Could you check a few things on this model? Use its own coordinates, in mm. Give positions to 0.01 mm unless a question says otherwise; leave off trailing zeros. Loops run counter-clockwise (first coordinate to the right, second up) from the corner with the lowest first, then second, coordinate; pieces in that order, holes last. Notation, with made-up numbers: (-33.5, 18.5) -> (11.5, 18.5) arc R26 ccw to (11.5, 54.5) -> close; hole circle Ø8 at (31.25, 5). An arc over 180 degrees is marked (long way). Put each result on its own line as item: value.
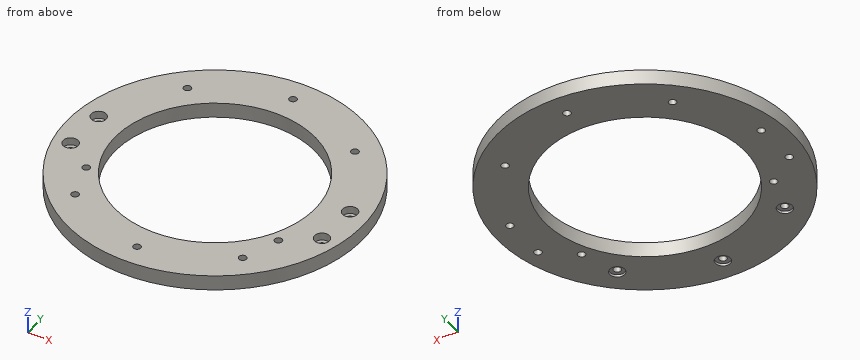
```python
from build123d import *

# Parameters (mm, degrees)
CYLINDER531_R     = 1.5
CYLINDER531_DEPTH = 100
CYLINDER530_R     = 1.5
CYLINDER530_DEPTH = 100
CYLINDER368_R     = 1.5
CYLINDER368_DEPTH = 50
CYLINDER369_R     = 3
CYLINDER369_DEPTH = 4
CYLINDER366_R     = 1.5
CYLINDER366_DEPTH = 50
CYLINDER358_R     = 1.5
CYLINDER358_DEPTH = 50
CYLINDER357_R     = 1.5
CYLINDER357_DEPTH = 50
CYLINDER361_R     = 3
CYLINDER361_DEPTH = 4
CYLINDER362_R     = 3
CYLINDER362_DEPTH = 4
CYLINDER332_R     = 3
CYLINDER332_DEPTH = 4
CYLINDER333_R     = 3
CYLINDER333_DEPTH = 4
CYLINDER352_R     = 3
CYLINDER352_DEPTH = 4
CYLINDER351_R     = 3
CYLINDER351_DEPTH = 4
CYLINDER344_R     = 1.5
CYLINDER344_DEPTH = 50
CYLINDER343_R     = 1.5
CYLINDER343_DEPTH = 50
CYLINDER340_R     = 1.5
CYLINDER340_DEPTH = 50
CYLINDER339_R     = 1.5
CYLINDER339_DEPTH = 50
CYLINDER338_R     = 1.5
CYLINDER338_DEPTH = 100
CYLINDER337_R     = 1.5
CYLINDER337_DEPTH = 100
CYLINDER301_R     = 1.5
CYLINDER301_DEPTH = 50
CYLINDER302_R     = 1.5
CYLINDER302_DEPTH = 50
TUBE018_R         = 59
TUBE018_R_2       = 40
TUBE018_DEPTH     = 6


with BuildPart() as obj1:
    # Cylinder531 → Cylinder531 (new body)
    with BuildSketch(Plane(origin=(39, -21, 0), x_dir=(1, 0, 0), z_dir=(0, 0, 1))):
        Circle(CYLINDER531_R)
    extrude(amount=CYLINDER531_DEPTH)


with BuildPart() as compound308:
    # Cylinder530 → Cylinder530 (new body)
    with BuildSketch(Plane(origin=(-39, -21, 0), x_dir=(1, 0, 0), z_dir=(0, 0, 1))):
        Circle(CYLINDER530_R)
    extrude(amount=CYLINDER530_DEPTH)

    # Compound308: union obj1
    add(obj1.part)


with BuildPart() as obj2:
    # Cylinder368 → Cylinder368 (new body)
    with BuildSketch(Plane(origin=(0, -50, 0), x_dir=(1, 0, 0), z_dir=(0, 0, 1))):
        Circle(CYLINDER368_R)
    extrude(amount=CYLINDER368_DEPTH)


with BuildPart() as obj3:
    # Cylinder369 → Cylinder369 (new body)
    with BuildSketch(Plane(origin=(0, -50, 9), x_dir=(1, 0, 0), z_dir=(0, 0, 1))):
        Circle(CYLINDER369_R)
    extrude(amount=CYLINDER369_DEPTH)


with BuildPart() as obj4:
    # Cylinder366 → Cylinder366 (new body)
    with BuildSketch(Plane(origin=(0, 50, 0), x_dir=(1, 0, 0), z_dir=(0, 0, 1))):
        Circle(CYLINDER366_R)
    extrude(amount=CYLINDER366_DEPTH)


with BuildPart() as obj5:
    # Cylinder358 → Cylinder358 (new body)
    with BuildSketch(Plane(origin=(-34, -36, 0), x_dir=(1, 0, 0), z_dir=(0, 0, 1))):
        Circle(CYLINDER358_R)
    extrude(amount=CYLINDER358_DEPTH)


with BuildPart() as compound306:
    # Cylinder357 → Cylinder357 (new body)
    with BuildSketch(Plane(origin=(34, -36, 0), x_dir=(1, 0, 0), z_dir=(0, 0, 1))):
        Circle(CYLINDER357_R)
    extrude(amount=CYLINDER357_DEPTH)

    # Compound306: union obj5
    add(obj5.part)


with BuildPart() as obj6:
    # Cylinder361 → Cylinder361 (new body)
    with BuildSketch(Plane(origin=(-34, -36, 0), x_dir=(1, 0, 0), z_dir=(0, 0, 1))):
        Circle(CYLINDER361_R)
    extrude(amount=CYLINDER361_DEPTH)


with BuildPart() as compound307:
    # Cylinder362 → Cylinder362 (new body)
    with BuildSketch(Plane(origin=(34, -36, 0), x_dir=(1, 0, 0), z_dir=(0, 0, 1))):
        Circle(CYLINDER362_R)
    extrude(amount=CYLINDER362_DEPTH)

    # Compound307: union obj6
    add(obj6.part)


with BuildPart() as compound307_1:
    # Compound307 placement: moved
    add(compound307.part.moved(Location((0, 0, 9))))


with BuildPart() as obj7:
    # Cylinder332 → Cylinder332 (new body)
    with BuildSketch(Plane(origin=(-51, 6, 17), x_dir=(1, 0, 0), z_dir=(0, 0, 1))):
        Circle(CYLINDER332_R)
    extrude(amount=CYLINDER332_DEPTH)


with BuildPart() as compound300:
    # Cylinder333 → Cylinder333 (new body)
    with BuildSketch(Plane(origin=(51, 6, 17), x_dir=(1, 0, 0), z_dir=(0, 0, 1))):
        Circle(CYLINDER333_R)
    extrude(amount=CYLINDER333_DEPTH)

    # Compound300: union obj7
    add(obj7.part)


with BuildPart() as compound300_1:
    # Compound300 placement: moved
    add(compound300.part.moved(Location((0, 0, -2))))


with BuildPart() as obj8:
    # Cylinder352 → Cylinder352 (new body)
    with BuildSketch(Plane(origin=(51, -12, 0), x_dir=(1, 0, 0), z_dir=(0, 0, 1))):
        Circle(CYLINDER352_R)
    extrude(amount=CYLINDER352_DEPTH)


with BuildPart() as compound303:
    # Cylinder351 → Cylinder351 (new body)
    with BuildSketch(Plane(origin=(-51, -12, 0), x_dir=(1, 0, 0), z_dir=(0, 0, 1))):
        Circle(CYLINDER351_R)
    extrude(amount=CYLINDER351_DEPTH)

    # Compound303: union obj8
    add(obj8.part)


with BuildPart() as compound303_1:
    # Compound303 placement: moved
    add(compound303.part.moved(Location((0, 0, 15))))


with BuildPart() as obj9:
    # Cylinder344 → Cylinder344 (new body)
    with BuildSketch(Plane(origin=(-34, 36, 0), x_dir=(1, 0, 0), z_dir=(0, 0, 1))):
        Circle(CYLINDER344_R)
    extrude(amount=CYLINDER344_DEPTH)


with BuildPart() as obj10:
    # Cylinder343 → Cylinder343 (new body)
    with BuildSketch(Plane(origin=(34, 36, 0), x_dir=(1, 0, 0), z_dir=(0, 0, 1))):
        Circle(CYLINDER343_R)
    extrude(amount=CYLINDER343_DEPTH)


with BuildPart() as obj11:
    # Cylinder340 → Cylinder340 (new body)
    with BuildSketch(Plane(origin=(51, 6, 0), x_dir=(1, 0, 0), z_dir=(0, 0, 1))):
        Circle(CYLINDER340_R)
    extrude(amount=CYLINDER340_DEPTH)


with BuildPart() as obj12:
    # Cylinder339 → Cylinder339 (new body)
    with BuildSketch(Plane(origin=(-51, 6, 0), x_dir=(1, 0, 0), z_dir=(0, 0, 1))):
        Circle(CYLINDER339_R)
    extrude(amount=CYLINDER339_DEPTH)


with BuildPart() as obj13:
    # Cylinder338 → Cylinder338 (new body)
    with BuildSketch(Plane(origin=(51, -12, 0), x_dir=(1, 0, 0), z_dir=(0, 0, 1))):
        Circle(CYLINDER338_R)
    extrude(amount=CYLINDER338_DEPTH)


with BuildPart() as compound301:
    # Cylinder337 → Cylinder337 (new body)
    with BuildSketch(Plane(origin=(-51, -12, 0), x_dir=(1, 0, 0), z_dir=(0, 0, 1))):
        Circle(CYLINDER337_R)
    extrude(amount=CYLINDER337_DEPTH)

    # Compound301: union obj9, obj10, obj11, obj12, obj13
    add(obj9.part)
    add(obj10.part)
    add(obj11.part)
    add(obj12.part)
    add(obj13.part)


with BuildPart() as obj14:
    # Cylinder301 → Cylinder301 (new body)
    with BuildSketch(Plane(origin=(34, 36, 0), x_dir=(1, 0, 0), z_dir=(0, 0, 1))):
        Circle(CYLINDER301_R)
    extrude(amount=CYLINDER301_DEPTH)


with BuildPart() as compound285:
    # Cylinder302 → Cylinder302 (new body)
    with BuildSketch(Plane(origin=(-34, 36, 0), x_dir=(1, 0, 0), z_dir=(0, 0, 1))):
        Circle(CYLINDER302_R)
    extrude(amount=CYLINDER302_DEPTH)

    # Compound285: union obj14
    add(obj14.part)


with BuildPart() as cut:
    # Tube018 → Tube018 (new body)
    with BuildSketch(Plane.XY.offset(12)):
        Circle(TUBE018_R)
        Circle(TUBE018_R_2, mode=Mode.SUBTRACT)
    extrude(amount=TUBE018_DEPTH)

    # Cut133: cut Compound285
    add(compound285.part, mode=Mode.SUBTRACT)

    # Cut145: cut Compound301
    add(compound301.part, mode=Mode.SUBTRACT)

    # Cut146: cut Compound303
    add(compound303_1.part, mode=Mode.SUBTRACT)

    # Cut147: cut Compound300
    add(compound300_1.part, mode=Mode.SUBTRACT)

    # Cut151: cut Compound307
    add(compound307_1.part, mode=Mode.SUBTRACT)

    # Cut152: cut Compound306
    add(compound306.part, mode=Mode.SUBTRACT)

    # Cut156: cut obj4
    add(obj4.part, mode=Mode.SUBTRACT)

    # Cut158: cut obj3
    add(obj3.part, mode=Mode.SUBTRACT)

    # Cut159: cut obj2
    add(obj2.part, mode=Mode.SUBTRACT)

    # Cut: cut Compound308
    add(compound308.part, mode=Mode.SUBTRACT)


solid = cut.part
```
1. If we section it at C-C (y = -21): List the corners of the cut face in (x, z) for me, then the cut area to 3 significant figures.
Recorded:
outline: (-55.14, 12) -> (-40.5, 12) -> (-40.5, 18) -> (-55.14, 18) -> close; (-37.5, 12) -> (-34.04, 12) -> (-34.04, 18) -> (-37.5, 18) -> close; (34.04, 12) -> (37.5, 12) -> (37.5, 18) -> (34.04, 18) -> close; (40.5, 12) -> (55.14, 12) -> (55.14, 18) -> (40.5, 18) -> close
area: 217 mm^2
2. I'm going to push flat-ended pins straight in: pin 1 (1.8 mm diameter, centred on x = -50, y = 6, fed in from +Z); pin 2 (1.8 mm diameter, centred on x = 34.5, y = -35.5, fed in from -Z); pin 3 (4 mm diameter, centred on x = 0, y = -50, fed in from +Z); pin 4 (3 mm diameter, centred on y = -41.5, z = 16.5, fed in from -X). Where does each tip first touch, or does it pass through?
Recorded:
pin 1: stops at z = 15
pin 2: stops at z = 13
pin 3: stops at z = 18
pin 4: stops at x = -43.37
3. I need wall thicknesses on line 1 (Y direction, x = 0, z = 12.55); line 2 (X direction, y = -1, z = 16.1); line 3 (Z direction, x = -1.5, y = -52). Which ranges of each line are inside material? Lowest first, please.
Recorded:
line 1: y = -59 to -53, -47 to -40, 40 to 48.5, 51.5 to 59
line 2: x = -58.99 to -39.99, 39.99 to 58.99
line 3: z = 13 to 18
4. If we section it at B-B (x = -20): List the corners of the cut face in (y, z) for me.
Recorded:
outline: (-55.51, 12) -> (-34.64, 12) -> (-34.64, 18) -> (-55.51, 18) -> close; (34.64, 12) -> (55.51, 12) -> (55.51, 18) -> (34.64, 18) -> close
5. If we section it at D-D (x = 34): List the corners of the cut face in (y, z) for me, then the cut area to 3 significant figures.
Recorded:
outline: (-48.22, 12) -> (-39, 12) -> (-39, 13) -> (-37.5, 13) -> (-37.5, 18) -> (-48.22, 18) -> close; (-34.5, 13) -> (-33, 13) -> (-33, 12) -> (-21.07, 12) -> (-21.07, 18) -> (-34.5, 18) -> close; (21.07, 12) -> (34.5, 12) -> (34.5, 18) -> (21.07, 18) -> close; (37.5, 12) -> (48.22, 12) -> (48.22, 18) -> (37.5, 18) -> close
area: 287 mm^2
6. If we section it at A-A (x = 0): List the corners of the cut face in (y, z) for me, then the cut area to 3 significant figures.
Recorded:
outline: (-59, 12) -> (-53, 12) -> (-53, 13) -> (-51.5, 13) -> (-51.5, 18) -> (-59, 18) -> close; (-48.5, 13) -> (-47, 13) -> (-47, 12) -> (-40, 12) -> (-40, 18) -> (-48.5, 18) -> close; (40, 12) -> (48.5, 12) -> (48.5, 18) -> (40, 18) -> close; (51.5, 12) -> (59, 12) -> (59, 18) -> (51.5, 18) -> close
area: 189 mm^2
